Can you work these out from the model? Positions are in its coordinate system, mm. A direction names the side the tool comes from. Give positions to 0.01 mm unless a question says otherwise; leave off trailing zeros. Loops run counter-clockwise (first coordinate to the right, second up) from the corner with the lowest first, then second, coordinate; pieces in that order, holes last. Notation, with made-up numbers: (-29, 28) -> (-5, 28) arc R16 ccw to (-5, 59) -> close; hole circle Ø11 at (39.25, 17.5). An arc over 180 degrees is marked (long way). Return JSON: item names as keys, results as strings. Group by question number.
Q1. Suppose I cut it at A-A, the plane z = 0. Please give me the cut outline in (x, y).
Q2. I need wall thicknesses on line 1 along X through (y, z) = (-1, 1.3); line 2 along X through (y, z) = (-3.5, -0.55). Which ranges of each line are inside material? Lowest first, please. Write a range as [from, to].
Q3. Will these pins go through, and if not, where does the flat tip stop? pin 1 (1.4 mm diameter, centred on y = -2.5, z = -0.5, fed in from -X); pin 2 (1.4 mm diameter, centred on y = -2.5, z = 0.5, fed in from +X); pin 3 (0.8 mm diameter, centred on x = -85.5, z = 0, fed in from -Y).
Q4. Which directions (+Z, -Z, +X, -X, +Y, -Y) give clear straight access to the entire face, cutting with the end or side of a thin tool? Please do faces 1 (the flat face through (81.111, -2, 0)), 2 (the flat face through (-83.911, -3, 0)), 3 (the flat face through (1, 0, -1.4)).
```python
from build123d import *

# Parameters (mm, degrees)
EXTRUDE_1_DEPTH = 1.4


with BuildPart() as part:
    # Эскиз1 → Бобышка-Вытянуть1 (new, symmetric)
    with BuildSketch(Plane.XY):
        Polygon((86.710588683, 0), (81.110588683, 0), (81.110588683, -3.92), (-83.910588683, -3.92), (-83.910588683, -1.12), (-86.710588683, -1.12), (-86.710588683, 3.92), (-43.02487952, 3.92), (86.710588683, 3.92), align=None)
    extrude(amount=EXTRUDE_1_DEPTH, both=True)


solid = part.part
```
Ans:
{
 "1": {"outline": "(-86.71, -1.12) -> (-83.91, -1.12) -> (-83.91, -3.92) -> (81.11, -3.92) -> (81.11, 0) -> (86.71, 0) -> (86.71, 3.92) -> (-86.71, 3.92) -> close"},
 "2": {"line 1": "x = [-86.71, 81.11]", "line 2": "x = [-83.91, 81.11]"},
 "3": {"pin 1": "stops at x = -83.91", "pin 2": "stops at x = 81.11", "pin 3": "stops at y = -1.12"},
 "4": {"face 1": "+Z, -Z, +X, -Y", "face 2": "+Z, -Z, -X, -Y", "face 3": "-Z, +X, -X, +Y, -Y"}
}
